from build123d import *

# Parameters (mm, degrees)
F1_DEPTH  = 3
F3_DEPTH  = 3
F5_DEPTH  = 2
F7_DEPTH  = 2
F8_R      = 1.5
F9_DEPTH  = 25
F10_R     = 4.5
F11_DEPTH = 25


with BuildPart() as f1:
    # F0 (on Top) → F1 (new body)
    with BuildSketch(Plane.XY):
        with BuildLine():
            Line((20, 0), (0, 0))
            Line((0, 0), (0, -29))
            ThreePointArc((0, -29), (0.87868, -31.12132), (3, -32))
            Line((3, -32), (17, -32))
            ThreePointArc((17, -32), (19.12132, -31.12132), (20, -29))
            Line((20, -29), (20, 0))
        make_face()
    extrude(amount=F1_DEPTH)

    # F2 (on face) → F3 (join)
    with BuildSketch(Plane(origin=(0, 0, 0), x_dir=(-1, 0, 0), z_dir=(0, 1, 0))):
        with BuildLine():
            Line((-20, 0), (0, 0))
            Line((0, 0), (0, 29))
            ThreePointArc((0, 29), (-0.87868, 31.12132), (-3, 32))
            Line((-3, 32), (-17, 32))
            ThreePointArc((-17, 32), (-19.12132, 31.12132), (-20, 29))
            Line((-20, 29), (-20, 0))
        make_face()
    extrude(amount=F3_DEPTH)

    # F4 (on face) → F5 (join)
    with BuildSketch(Plane(origin=(0, 0, 0), x_dir=(0, -1, 0), z_dir=(-1, 0, 0))):
        Polygon((29, 3), (0, 29), (0, 3), align=None)
    extrude(amount=-F5_DEPTH)

    # F6 (on face) → F7 (join)
    with BuildSketch(Plane.YZ.offset(20)):
        Polygon((0, 3), (0, 29), (-29, 3), align=None)
    extrude(amount=-F7_DEPTH)

    # F8 (on face) → F9 (cut)
    with BuildSketch(Plane.XY.offset(3)):
        with Locations((10, -21.589138)):
            Circle(F8_R)
    extrude(amount=-F9_DEPTH, mode=Mode.SUBTRACT)

    # F10 (on face) → F11 (cut)
    with BuildSketch(Plane.XZ):
        with Locations((10, 23)):
            Circle(F10_R)
    extrude(amount=-F11_DEPTH, mode=Mode.SUBTRACT)


solid = f1.part
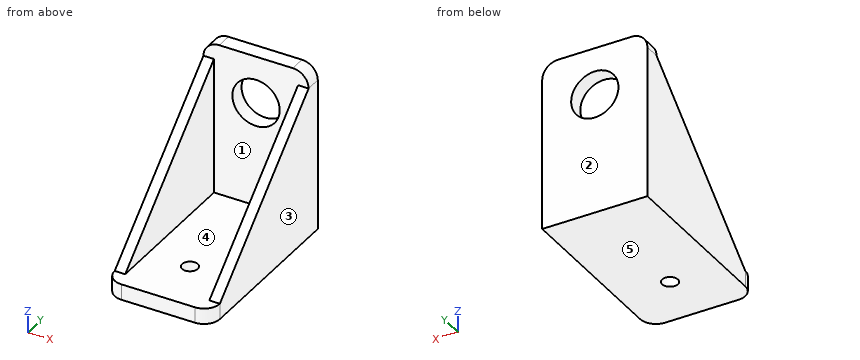
The model under review builds one solid part; all positions refer to its coordinate system, in mm. Face numbers are marked on the shaded views. A direction names the side the tool comes from. Give positions to 0.01 mm unless a question says otherwise; leave off trailing zeros. Write each loop counter-clockwise with the first axis right and the second up, starting at its lowest first coordinate (ties: lowest second). Pieces come first, ordered by that corner, then holes. Notation, with made-up numbers: M 19.25,19 L 59.25,19 A15 ccw 59.25,36 Z; hole C 9,-31 d4. An arc over 180 degrees is marked long. One line per question, with ' | ' between items. Start each with the question number.
Item 1: For the marked faces 4 and 5, list the 3-axis set-ups (+Z, -Z, +X, -X, +Y, -Y) from which the entire face can be reached by the end or side of a thin tool; tool diameter is ignored.
Item 2: We need section A-A on x = 10. Write out the cut boundary in (y, z).
Item 3: For pin 1 (6 mm diameter, centred on x = 14, y = -20, fed in from +Z); pin 2 (8 mm diameter, centred on x = 17, y = -24, fed in from +Z); pin 3 (1 mm diameter, centred on x = 11, z = 10.5, fed in from -Y), all flat-tipped, find the tip position at first contact; note any pin that passes through.
Item 4: We need section C-C on y = -14.5. Write out the cut boundary in (x, z).
Item 5: We need section D-D on z = 11. Write out the cut boundary in (x, y).
Item 6: Wall thickness on line 1 (X direction, y = -8.5, z = 14); line 2 (Y direction, x = 10, z = 2.15); line 3 (Y direction, x = 10.5, z = 13): over which ranges is each line inside the solid? List them lowest first. Write a range as from..to.
Item 7: Draft analysis for pull direction X (two halves, no side actions). For the marked faces 1, 2 and 3, state which applies: released by +X, released by -X, zero draft, split by the parting line, or undercut.
Item 8: We need section B-B on z = 23. Write out the cut boundary in (x, y).
Results found:
1) face 4: +Z, -Y | face 5: -Z, +X, -X, +Y, -Y
2) outline: M -32,0 L -23.09,0 L -23.09,3 L -32,3 Z; M -20.09,0 L 3,0 L 3,18.5 L 0,18.5 L 0,3 L -20.09,3 Z; M 0,27.5 L 3,27.5 L 3,32 L 0,32 Z
3) pin 1: stops at z = 3 | pin 2: stops at z = 10.96 | pin 3: stops at y = 0
4) outline: M 0,0 L 20,0 L 20,16 L 18,16 L 18,3 L 2,3 L 2,16 L 0,16 Z
5) outline: M 0,-20.08 L 2,-20.08 L 2,0 L 18,0 L 18,-20.08 L 20,-20.08 L 20,3 L 0,3 Z
6) line 1: x = 0..2, 18..20 | line 2: y = -32..-23.09, -20.09..3 | line 3: y = 0..3
7) face 1: undercut | face 2: zero draft | face 3: released by +X
8) outline: M 0,-6.69 L 2,-6.69 L 2,0 L 5.5,0 L 5.5,3 L 0,3 Z; M 14.5,0 L 18,0 L 18,-6.69 L 20,-6.69 L 20,3 L 14.5,3 Z
